Build history of the part. All positions in model axes, mm. Face numbers are marked on the shaded views. A direction names the side the tool comes from. Give positions to 0.01 mm unless a question says otherwise; leave off trailing zeros. Write each loop counter-clockwise with the first axis right and the second up, starting at its lowest first coordinate (ties: lowest second). Pieces come first, ordered by that corner, then holes. Notation, with made-up numbers: (-12, 9) -> (-7, 9) arc R24 ccw to (-7, 33) -> close; hole circle Ø3 at (-32, -9.75). An arc over 180 degrees is marked (long way). One line per question, with ' | ' between items. Start each with the question number.
(1) Drill centre lines: probe 1 along X at (y, z) = (1.85, -8.5); probe 2 along Y at (x, z) = (3.5, -1); probe 3 along Z at (x, y) = (15, 9.75). Where is each one in solid material? Low to high. Write a range as from..to.
(2) Tool access for the marked faces 5 and 6: list every direction of +Z, -Z, +X, -X, +Y, -Y with a clear straight run to the whole face (end or side of a thin tool).
(3) Band-saw the part on C-C, the plane x = 5. Give the cut face in (y, z), and give its area (3 significant figures).
(4) Band-saw the part on B-B, the plane y = 10. Give the cut face in (x, z).
(5) Band-saw the part on A-A, the plane z = -8.5. Give the cut face in (x, y), and give its area (4 significant figures).
(6) Pin check, flat tips, straight feed: P1, Ø2, axis at x = 7, y = 4, coming from the +Z side; P2, Ø7, axis at x = 4.5, z = -10.5, coming from the +Y side; P3, Ø4.5, axis at x = 8.5, y = 10, coming from the +Z side; P4, Ø1.5, axis at x = 15, z = -15.5, coming from the -Y side. Stop position of each tip, or through.
(7) Band-saw the part on D-D, the plane x = 8.5. Give the cut face in (y, z).
(8) Pull direction Z, two halves, no side cores. Call the marked faces 1, 2, 3 and 4: released by +Z, released by -Z, zero draft, split by the parting line, or undercut.
from build123d import *

# Parameters (mm, degrees)
EXTRUDE_1_DEPTH     = 17
FILLET_1_R          = 2.5
SKETCH_2_R          = 2.55
CUT_EXTRUDE_1_DEPTH = 17
SKETCH_3_R          = 2.55
CUT_EXTRUDE_2_DEPTH = 17


with BuildPart() as part:
    # Эскиз1 → Бобышка-Вытянуть1 (new body)
    with BuildSketch(Plane(origin=(0, 0, 0), x_dir=(0, 0, -1), z_dir=(1, 0, 0))):
        with BuildLine():
            Line((14, 2.5), (0, 2.5))
            Line((0, 2.5), (0, 0))
            Line((0, 0), (14, 0))
            ThreePointArc((14, 0), (17.181980515, 1.318019485), (18.5, 4.5))
            Line((18.5, 4.5), (18.5, 18.5))
            Line((18.5, 18.5), (16, 18.5))
            Line((16, 18.5), (16, 4.5))
            ThreePointArc((16, 4.5), (15.414213562, 3.085786438), (14, 2.5))
        make_face()
    extrude(amount=EXTRUDE_1_DEPTH)

    # Скругление1
    fillet_1_edges = [part.edges().sort_by_distance(p)[0] for p in [
        (0, 1.25, 0),
        (17, 18.5, -17.25),
        (17, 1.25, 0),
        (0, 18.5, -17.25),
    ]]
    fillet(fillet_1_edges, radius=FILLET_1_R)

    # Эскиз2 → Вырез-Вытянуть1 (cut)
    with BuildSketch(Plane.XZ):
        with Locations(Location((8.5, -8.5, 0), (0, 0, 270))):
            Circle(SKETCH_2_R)
    extrude(amount=-CUT_EXTRUDE_1_DEPTH, mode=Mode.SUBTRACT)

    # Эскиз3 → Вырез-Вытянуть2 (cut)
    with BuildSketch(Plane(origin=(0, 0, -18.5), x_dir=(-1, 0, 0), z_dir=(0, 0, -1))):
        with Locations((-8.5, 10)):
            Circle(SKETCH_3_R)
    extrude(amount=-CUT_EXTRUDE_2_DEPTH, mode=Mode.SUBTRACT)


solid = part.part
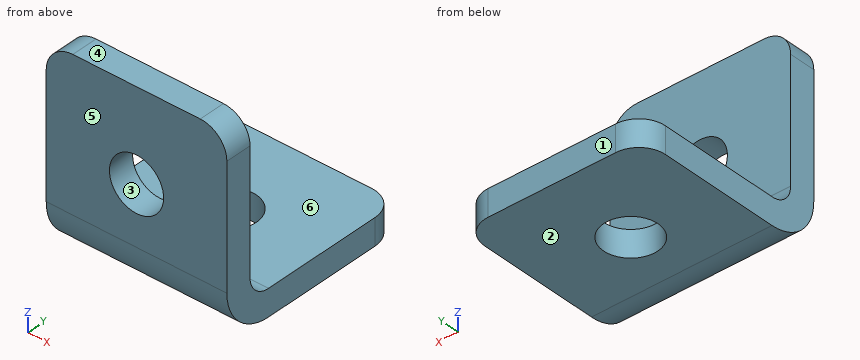
Results:
1) probe 1: x = 0..5.95, 11.05..17 | probe 2: y = 0..2.5 | probe 3: z = -18.5..-16
2) face 5: +Z, -Z, +X, -X, -Y | face 6: +Z, +X, -X, +Y
3) outline: (0, -14) arc R4.5 ccw to (4.5, -18.5) -> (18.5, -18.5) -> (18.5, -16) -> (4.5, -16) arc R2 cw to (2.5, -14) -> (2.5, 0) -> (0, 0) -> close | area: 82.8 mm²
4) outline: (0, -18.5) -> (5.95, -18.5) -> (5.95, -16) -> (0, -16) -> close; (11.05, -18.5) -> (17, -18.5) -> (17, -16) -> (11.05, -16) -> close
5) outline: (0, 0) -> (5.95, 0) -> (5.95, 2.5) -> (0, 2.5) -> close; (11.05, 0) -> (17, 0) -> (17, 2.5) -> (11.05, 2.5) -> close | area: 29.75 mm²
6) P1: stops at z = -15.32 | P2: stops at y = 2.5 | P3: passes through | P4: stops at y = 0.06
7) outline: (0, -14) arc R4.5 ccw to (4.5, -18.5) -> (7.45, -18.5) -> (7.45, -16) -> (4.5, -16) arc R2 cw to (2.5, -14) -> (2.5, -11.05) -> (0, -11.05) -> close; (0, -5.95) -> (2.5, -5.95) -> (2.5, 0) -> (0, 0) -> close; (12.55, -18.5) -> (18.5, -18.5) -> (18.5, -16) -> (12.55, -16) -> close
8) face 1: zero draft | face 2: released by -Z | face 3: undercut | face 4: released by +Z
